Can you work these out from the model? Positions are in its coordinate system, mm. Face numbers are marked on the shaded views. A direction names the side the tool comes from. Give positions to 0.01 mm unless a question says otherwise; leave off trailing zeros. Loops run counter-clockwise (first coordinate to the right, second up) from the corner with the lowest first, then second, coordinate; pieces in that order, holes last. Notation, with made-up numbers: (34.5, 59.25) -> (78.5, 59.25) arc R32 cw to (78.5, 97.25) -> close; hole circle Ø11 at (37.25, -7.5). An arc over 180 degrees is marked (long way). One line per question, with ' | ' between items.
from build123d import *

# Parameters (mm, degrees)
SKETCH1_W           = 50
SKETCH1_H           = 50
BOSS_EXTRUDE1_DEPTH = 5
CUT_EXTRUDE1_DEPTH  = 71.887234394


with BuildPart() as part:
    # Sketch1 → Boss-Extrude1 (new body)
    with BuildSketch(Plane.XY):
        with Locations((25, 25)):
            Rectangle(SKETCH1_W, SKETCH1_H)
    extrude(amount=BOSS_EXTRUDE1_DEPTH)

    # Sketch2 → Cut-Extrude1 (cut, through all)
    with BuildSketch(Plane.XY.offset(5)):
        with BuildLine():
            Line((10.1, 43), (10.1, 7))
            ThreePointArc((10.1, 7), (13.1, 4), (16.1, 7))
            Line((16.1, 7), (16.1, 43))
            ThreePointArc((16.1, 43), (13.1, 46), (10.1, 43))
        make_face()
        with BuildLine():
            Line((33.9, 43), (33.9, 7))
            ThreePointArc((33.9, 7), (36.9, 4), (39.9, 7))
            Line((39.9, 7), (39.9, 43))
            ThreePointArc((39.9, 43), (36.9, 46), (33.9, 43))
        make_face()
    extrude(amount=-CUT_EXTRUDE1_DEPTH, mode=Mode.SUBTRACT)


solid = part.part
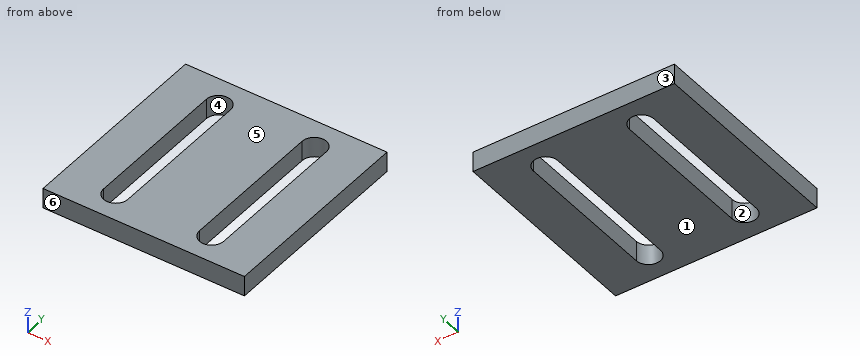
Q1. If we section it at B-B (x = 13.1): Write out the boundary of the cut face in (y, z).
Entries:
outline: (0, 0) -> (4, 0) -> (4, 5) -> (0, 5) -> close; (46, 0) -> (50, 0) -> (50, 5) -> (46, 5) -> close
Q2. On a 3-axis mill with a long thin cutter (end or side, diameter ignored), from which of +Z, -Z, +X, -X, +Y, -Y can I reach the whole of each face in a straight line? I mean the marked faces 1 and 2. Say none if no direction works.
Entries:
face 1: -Z, +X, -X, +Y, -Y | face 2: +Z, -Z
Q3. If we mould it in two halves opening along Y, with no side actions, what happens to the marked faces 3, 4, 5 and 6? For each: pulls with the +Y half, pulls with the -Y half, needs draft (parallel to the pull), parting line crosses it, or undercut.
Entries:
face 3: pulls with the +Y half | face 4: undercut | face 5: needs draft | face 6: pulls with the -Y half
Q4. If we section it at C-C (z = 1.65): Write out the boundary of the cut face in (x, y), plus the area to 3 significant figures.
Entries:
outline: (0, 0) -> (50, 0) -> (50, 50) -> (0, 50) -> close; hole (10.1, 7) arc R3 ccw to (16.1, 7) -> (16.1, 43) arc R3 ccw to (10.1, 43) -> close; hole (33.9, 7) arc R3 ccw to (39.9, 7) -> (39.9, 43) arc R3 ccw to (33.9, 43) -> close | area: 2,010 mm²
Q5. If we section it at A-A (y = 39): Write out the boundary of the cut face in (x, z).
Entries:
outline: (0, 0) -> (10.1, 0) -> (10.1, 5) -> (0, 5) -> close; (16.1, 0) -> (33.9, 0) -> (33.9, 5) -> (16.1, 5) -> close; (39.9, 0) -> (50, 0) -> (50, 5) -> (39.9, 5) -> close
Q6. If I drill on probe 1 along X at (y, z) = (29, 3.15); probe 2 along X at (y, z) = (45, 2.1); probe 3 along Y at (x, z) = (13, 4.1), over which ranges is the centre line in solid material (lowest first)? Write a range as from..to.
Entries:
probe 1: 0..10.1, 16.1..33.9, 39.9..50 | probe 2: 0..10.86, 15.34..34.66, 39.14..50 | probe 3: 0..4, 46..50
Q7. If we section it at D-D (y = 45): Write out the boundary of the cut face in (x, z).
Entries:
outline: (0, 0) -> (10.86, 0) -> (10.86, 5) -> (0, 5) -> close; (15.34, 0) -> (34.66, 0) -> (34.66, 5) -> (15.34, 5) -> close; (39.14, 0) -> (50, 0) -> (50, 5) -> (39.14, 5) -> close
